CAD build for the part. Positions are in the model's coordinates, mm. Face numbers are marked on the shaded views. A direction names the side the tool comes from. Coordinates: 2 decimals unless noted, no trailing zeros. Order: outer loops, then holes, each group sorted by start corner. A loop starts at its lowest first (then second) coordinate and runs counter-clockwise, first axis right, second up. Notation, with made-up numbers: M 18,43 L 74,43 A25 ccw 74,68 Z; hole C -29.75,67 d6. An arc over 180 degrees is marked long. Write item = value, one per line.
from build123d import *

# Parameters (mm, degrees)
SKETCH_2_W          = 75
SKETCH_2_H          = 45
EXTRUDE_3_DEPTH     = 8
SKETCH_5_W          = 70.2
SKETCH_5_H          = 40.2
CUT_EXTRUDE_1_DEPTH = 1.8
SKETCH_7_R          = 1.5
CUT_EXTRUDE_4_DEPTH = 2.2
SKETCH_8_W          = 15
SKETCH_8_H          = 10
SKETCH_8_W_2        = 10
SKETCH_8_H_2        = 15
SKETCH_8_H_3        = 12
CUT_EXTRUDE_6_DEPTH = 3


with BuildPart() as part:
    # 草图2 → 凸台-拉伸3 (new body)
    with BuildSketch(Plane(origin=(0, 0, 0), x_dir=(1, 0, 0), z_dir=(0, 1, 0))):
        with Locations((37.5, 22.5)):
            Rectangle(SKETCH_2_W, SKETCH_2_H)
    extrude(amount=EXTRUDE_3_DEPTH)

    # 草图5 → 切除-拉伸1 (cut)
    with BuildSketch(Plane(origin=(0, 8, 0), x_dir=(1, 0, 0), z_dir=(0, 1, 0))):
        with Locations((37.5, 22.5)):
            Rectangle(SKETCH_5_W, SKETCH_5_H)
    extrude(amount=-CUT_EXTRUDE_1_DEPTH, mode=Mode.SUBTRACT)

    # 草图7 → 切除-拉伸4 (cut)
    with BuildSketch(Plane(origin=(0, 6.2, 0), x_dir=(1, 0, 0), z_dir=(0, 1, 0))):
        with Locations(Location((7.4, 37.6, 0), (0, 0, 270))):
            Circle(SKETCH_7_R)
        with Locations(Location((67.6, 37.6, 0), (0, 0, 90))):
            Circle(SKETCH_7_R)
        with Locations(Location((7.4, 7.4, 0), (0, 0, 90))):
            Circle(SKETCH_7_R)
        with Locations(Location((67.6, 7.4, 0), (0, 0, 270))):
            Circle(SKETCH_7_R)
    extrude(amount=-CUT_EXTRUDE_4_DEPTH, mode=Mode.SUBTRACT)

    # 草图8 → 切除-拉伸6 (cut)
    with BuildSketch(Plane(origin=(0, 6.2, 0), x_dir=(1, 0, 0), z_dir=(0, 1, 0))):
        with Locations((19.9, 9.4)):
            Rectangle(SKETCH_8_W, SKETCH_8_H)
        with Locations((65.6, 25.1)):
            Rectangle(SKETCH_8_W_2, SKETCH_8_H_2)
        with Locations((34.9, 33.6)):
            Rectangle(SKETCH_8_W, SKETCH_8_H_3)
    extrude(amount=-CUT_EXTRUDE_6_DEPTH, mode=Mode.SUBTRACT)


solid = part.part
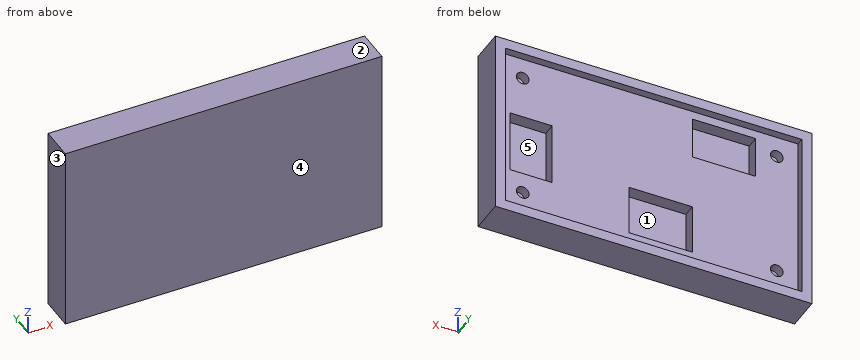
(1) Wall check: line 1 (X direction, y = 4.7, z = -37.6); line 2 (Z direction, x = 67.6, y = 5.6); line 3 (Z direction, x = 30, y = 5.25). Give the ranges that are in metal, low to high. Write a range as from..to.
Evaluation:
line_1 = 0..5.9, 8.9..27.4, 42.4..66.1, 69.1..75
line_2 = -45..-39.1, -36.1..-32.6, -17.6..-8.9, -5.9..0
line_3 = -45..-39.6, -27.6..0
(2) Slice it at D-D, the plane x = 37.5. Write the cut outline in (y, z), then the cut area to 3 significant figures.
Evaluation:
outline = M 0,-45 L 8,-45 L 8,-42.6 L 6.2,-42.6 L 6.2,-39.6 L 3.2,-39.6 L 3.2,-27.6 L 6.2,-27.6 L 6.2,-2.4 L 8,-2.4 L 8,0 L 0,0 Z
area = 252 mm²
(3) Pin check, flat tips, straight feed: pin 1 Ø3.5 at (x, z) = (7.4, -37.6) entering from +Y; pin 2 Ø0.9 at (x, z) = (68, -7.5) entering from +Y. Stop position of each tip, or through.
Evaluation:
pin_1 = 6.2
pin_2 = 4
(4) Pull direction X, two halves, no side cores. Call the marked faces 3, 4 and 5: +X half, -X half, draft (parallel to the pull), parting line (faces both ways), or undercut.
Evaluation:
face_3 = -X half
face_4 = draft
face_5 = undercut
(5) Slice it at C-C, the plane z = -37.6. Write the cut outline in (x, y), then the cut area to 3 significant figures.
Evaluation:
outline = M 0,0 L 75,0 L 75,8 L 72.6,8 L 72.6,6.2 L 69.1,6.2 L 69.1,4 L 66.1,4 L 66.1,6.2 L 42.4,6.2 L 42.4,3.2 L 27.4,3.2 L 27.4,6.2 L 8.9,6.2 L 8.9,4 L 5.9,4 L 5.9,6.2 L 2.4,6.2 L 2.4,8 L 0,8 Z
area = 415 mm²
(6) Slice it at B-B, the plane x = 22.5. Write the cut outline in (y, z).
Evaluation:
outline = M 0,-45 L 8,-45 L 8,-42.6 L 6.2,-42.6 L 6.2,-14.4 L 3.2,-14.4 L 3.2,-4.4 L 6.2,-4.4 L 6.2,-2.4 L 8,-2.4 L 8,0 L 0,0 Z
(7) Slice it at A-A, the plane y = 5.25. Write the cut outline in (x, z), then the cut area to 3 significant figures.
Evaluation:
outline = M 0,-45 L 75,-45 L 75,0 L 0,0 Z; hole C 7.4,-37.6 d3; hole C 7.4,-7.4 d3; hole M 12.4,-14.4 L 27.4,-14.4 L 27.4,-4.4 L 12.4,-4.4 Z; hole M 27.4,-39.6 L 42.4,-39.6 L 42.4,-27.6 L 27.4,-27.6 Z; hole M 60.6,-32.6 L 70.6,-32.6 L 70.6,-17.6 L 60.6,-17.6 Z; hole C 67.6,-37.6 d3; hole C 67.6,-7.4 d3
area = 2,870 mm²
(8) Tool access for the marked faces 1 and 2: list every direction of +Z, -Z, +X, -X, +Y, -Y with a clear straight run to the whole face (end or side of a thin tool).
Evaluation:
face_1 = +Y
face_2 = +Z, +X, -X, +Y, -Y
